CAD build for the part. Positions are in the model's coordinates, mm. A direction names the side the tool comes from. Round coordinates to 2 decimals unless told otherwise and drop trailing zeros. Order: outer loops, then holes, each group sorted by start corner. A loop starts at its lowest first (then second) coordinate and runs counter-clockwise, first axis right, second up. Notation, with made-up numbers: M -38,79 L 11,79 A24 ccw 11,91 Z; hole C -34,2 d5. An arc over 180 degrees is marked long. Answer as a JSON object with one key per item and string values.
```python
from build123d import *

# Parameters (mm, degrees)
PAD002_DEPTH = 3.3
PAD_DEPTH    = 0.7
PAD001_DEPTH = 9.42
FILLET_R     = 0.75
SKETCH002_R  = 1.6
POCKET_DEPTH = 2.5


with BuildPart() as body001:
    # Sketch003 (on Face1 of ReferencePocket) → Pad002 (new body)
    with BuildSketch(Plane(origin=(0, 0, 0), x_dir=(1, 0, 0), z_dir=(0, 0, -1))):
        with BuildLine():
            Line((-7.755, 3.575), (-7.485, 3.575))
            ThreePointArc((-7.485, 3.575), (-7.414289, 3.604289), (-7.385, 3.675))
            Line((-7.385, 3.675), (-7.385, 3.945))
            ThreePointArc((-7.385, 3.945), (-7.414289, 4.015711), (-7.485, 4.045))
            Line((-7.485, 4.045), (-7.755, 4.045))
            ThreePointArc((-7.755, 4.045), (-7.825711, 4.015711), (-7.855, 3.945))
            Line((-7.855, 3.945), (-7.855, 3.675))
            ThreePointArc((-7.855, 3.675), (-7.825711, 3.604289), (-7.755, 3.575))
        make_face()
    extrude(amount=PAD002_DEPTH)


with BuildPart() as fusion:
    # Clone base: copy of Body001
    add(body001.part)


with BuildPart() as fusion_1:
    # Clone placement: moved
    add(fusion.part.moved(Location((0, 7.62, 0))))

    # Fusion: union Body001
    add(body001.part)


with BuildPart() as fusion001:
    # Clone001 base: copy of Fusion
    add(fusion_1.part)


with BuildPart() as fusion001_1:
    # Clone001 placement: moved
    add(fusion001.part.moved(Location((2.54, 0, 0))))


with BuildPart() as fusion002:
    # Clone002 base: copy of Fusion
    add(fusion_1.part)


with BuildPart() as fusion002_1:
    # Clone002 placement: moved
    add(fusion002.part.moved(Location((10.16, 0, 0))))


with BuildPart() as fusion003:
    # Clone003 base: copy of Fusion
    add(fusion_1.part)


with BuildPart() as fusion003_1:
    # Clone003 placement: moved
    add(fusion003.part.moved(Location((12.7, 0, 0))))


with BuildPart() as fusion004:
    # Clone004 base: copy of Fusion
    add(fusion_1.part)


with BuildPart() as fusion004_1:
    # Clone004 placement: moved
    add(fusion004.part.moved(Location((15.24, 0, 0))))


with BuildPart() as fusion005:
    # Fusion001 base: copy of Fusion
    add(fusion_1.part)

    # Fusion001: union Fusion001, Fusion002, Fusion003, Fusion004
    add(fusion001_1.part)
    add(fusion002_1.part)
    add(fusion003_1.part)
    add(fusion004_1.part)


with BuildPart() as fusion006:
    # Sketch → Pad (new body)
    with BuildSketch(Plane.XY):
        with BuildLine():
            Line((-10.06, -6.25), (8.006793, -6.25))
            ThreePointArc((8.006793, -6.25), (9.45863, -5.64863), (10.06, -4.196793))
            Line((10.06, -4.196793), (10.06, 4.196793))
            ThreePointArc((10.06, 4.196793), (9.45863, 5.64863), (8.006793, 6.25))
            Line((8.006793, 6.25), (-8.006793, 6.25))
            ThreePointArc((-8.006793, 6.25), (-9.45863, 5.64863), (-10.06, 4.196793))
            Line((-10.06, 4.196793), (-10.06, -6.25))
        make_face()
    extrude(amount=PAD_DEPTH)

    # Sketch001 (on Face9 of Pad) → Pad001 (join)
    with BuildSketch(Plane.XY.offset(0.7)):
        with BuildLine():
            Line((-9.265, -5.455), (7.830229, -5.455))
            ThreePointArc((7.830229, -5.455), (8.844765, -5.034765), (9.265, -4.020229))
            Line((9.265, -4.020229), (9.265, 4.020228))
            ThreePointArc((9.265, 4.020228), (8.844765, 5.034765), (7.830229, 5.455))
            Line((7.830229, 5.455), (-7.830229, 5.455))
            ThreePointArc((-7.830229, 5.455), (-8.844765, 5.034765), (-9.265, 4.020228))
            Line((-9.265, 4.020228), (-9.265, -5.455))
        make_face()
    extrude(amount=PAD001_DEPTH)

    # Fillet
    fillet_edges = [fusion006.edges().sort_by_distance(p)[0] for p in [
        (-0.717386, -5.455, 0.7),
        (8.844765, -5.034765, 0.7),
        (9.265, 0, 0.7),
        (8.844765, 5.034765, 0.7),
        (0, 5.455, 0.7),
        (-8.844765, 5.034765, 0.7),
        (-9.265, -0.717386, 0.7),
        (-9.265, -0.717386, 10.12),
        (-8.844765, 5.034765, 10.12),
        (0, 5.455, 10.12),
        (8.844765, 5.034765, 10.12),
        (9.265, 0, 10.12),
        (8.844765, -5.034765, 10.12),
        (-0.717386, -5.455, 10.12),
    ]]
    fillet(fillet_edges, radius=FILLET_R)

    # Sketch002 (on Face31 of Fillet) → Pocket (cut)
    with BuildSketch(Plane.XY.offset(10.12)):
        with Locations((0.5, 0)):
            Circle(SKETCH002_R)
    extrude(amount=-POCKET_DEPTH, mode=Mode.SUBTRACT)

    # Fusion002: union Fusion005
    add(fusion005.part)


solid = fusion006.part
```
Item 1: Wall check: line 1 along Y through (x, z) = (0.5, 9.1) (3 decimals); line 2 along X through (y, z) = (4, -2.5); line 3 along Z through (x, y) = (8, -1.75). Give the ranges that are in metal, low to high. Write a range as [from, to].
Worked answers:
{"line 1": "y = [-5.455, -1.6], [1.6, 5.455]", "line 2": "x = [-7.84, -7.4], [-5.3, -4.86], [2.32, 2.76], [4.86, 5.3], [7.4, 7.84]", "line 3": "z = [0, 10.12]"}
Item 2: Saw through at C-C on x = 0.5. List the corners of the cut face in (y, z) (3 decimals).
Worked answers:
{"outline": "M -6.25,0 L 6.25,0 L 6.25,0.7 L 6.205,0.7 A0.75 cw 5.455,1.45 L 5.455,9.37 A0.75 ccw 4.705,10.12 L 1.6,10.12 L 1.6,7.62 L -1.6,7.62 L -1.6,10.12 L -4.705,10.12 A0.75 ccw -5.455,9.37 L -5.455,1.45 A0.75 cw -6.205,0.7 L -6.25,0.7 Z"}
Item 3: Two-plate mould, pull along X, no slides. Class faces 6 (the flat face through (-9.265, -1, 5)), 7 (the cylindrical face through (2.026, 0.481, 8.888)), 8 (the cylindrical face through (9.443, -5.665, 0.345)): released by +X, released by -X, zero draft, split by the parting line, or undercut.
Worked answers:
{"face 6": "released by -X", "face 7": "undercut", "face 8": "released by +X"}
Item 4: 3-axis set-ups, long thin cutter, end or side, ignore diameter. For faces 1 (the flat face through (-1, -5.455, 5)), 2 (the flat face through (0, 0, 7.62)), 3 (the flat face through (9.265, 0, 5)), 4 (the flat face through (0, 5.455, 5)), 5 (the cylindrical face through (8.83, -5.05, 5.35)): which of +Z, -Z, +X, -X, +Y, -Y reach the whole face in a straight line?
Worked answers:
{"face 1": "+Z, +X, -X, -Y", "face 2": "+Z", "face 3": "+Z, +X, +Y, -Y", "face 4": "+Z, +X, -X, +Y", "face 5": "+Z, +X, -Y"}
Item 5: Drop flat-ended pins along their axis: pin 1 Ø3 at (y, z) = (-5, 5) entering from +X (3 decimals); pin 2 Ø1.5 at (x, y) = (0.5, 1.5) entering from -Z; pin 3 Ø2 at (x, z) = (-5.5, 3.5) entering from +Y (3 decimals). Give the stop position or say it passes through.
Worked answers:
{"pin 1": "stops at x = 9.265", "pin 2": "stops at z = 0", "pin 3": "stops at y = 5.455"}
Item 6: Saw through at B-B on y = 0. List the corners of the cut face in (x, z) (3 decimals), and give its area (3 significant figures).
Worked answers:
{"outline": "M -10.06,0 L 10.06,0 L 10.06,0.7 L 10.015,0.7 A0.75 cw 9.265,1.45 L 9.265,9.37 A0.75 ccw 8.515,10.12 L 2.1,10.12 L 2.1,7.62 L -1.1,7.62 L -1.1,10.12 L -8.515,10.12 A0.75 ccw -9.265,9.37 L -9.265,1.45 A0.75 cw -10.015,0.7 L -10.06,0.7 Z", "area": "181 mm2"}
Item 7: Saw through at D-D on y = -2.5. List the corners of the cut face in (x, z) (3 decimals).
Worked answers:
{"outline": "M -10.06,0 L 10.06,0 L 10.06,0.7 L 10.015,0.7 A0.75 cw 9.265,1.45 L 9.265,9.37 A0.75 ccw 8.515,10.12 L -8.515,10.12 A0.75 ccw -9.265,9.37 L -9.265,1.45 A0.75 cw -10.015,0.7 L -10.06,0.7 Z"}
Item 8: Saw through at A-A on z = 4.75. List the corners of the cut face in (x, y) (3 decimals).
Worked answers:
{"outline": "M -9.265,-5.455 L 7.83,-5.455 A1.435 ccw 9.265,-4.02 L 9.265,4.02 A1.435 ccw 7.83,5.455 L -7.83,5.455 A1.435 ccw -9.265,4.02 Z"}
